Geometry check sheet. Reference: the model listing, model coordinates, mm. Give positions to 0.01 mm unless a question says otherwise; leave off trailing zeros. Loops run counter-clockwise (first coordinate to the right, second up) from the corner with the lowest first, then second, coordinate; pieces in that order, holes last.
1. Cross-section at D-D, the plane z = 76.5. Record the cut outline in (x, y).
2. Release check for a two-part mould opening along X. For faces 1 (the flat face through (64, 0, 54)), 2 (the cylindrical face through (36.71, 2.46, 91.41)), 3 (the flat face through (65.6, 2.5, -8.5)), 4 (the cylindrical face through (72.68, 2.54, 40.54)) record: +X half, -X half, draft (parallel to the pull), parting line (faces both ways), or undercut.
3. Go/stop test with flat-tipped pins: pin 1 Ø1.5 at (y, z) = (4, 19) entering from +X; pin 2 Ø3 at (x, y) = (39, 3.5) entering from +Z; pin 3 Ø3 at (x, y) = (58.5, 3.5) entering from +Z. Record where each tip stops, or that it passes through.
4. Cross-section at B-B, the plane x = 63.5. Record the cut outline in (y, z), plus the area to 3 significant figures.
5. Material ranges on L1, parallel to X at y = 3.7, z = 46.5; L2, parallel to X at y = 0.55, z = 43; L3, parallel to Z at x = 58, y = 3.75, recorded low to high.
6. Cross-section at C-C, the plane y = 2.35. Record the cut outline in (x, z), plus the area to 3 significant figures.
7. Cross-section at A-A, the plane z = 48. Record the cut outline in (x, y), plus the area to 3 significant figures.
from build123d import *

# Parameters (mm, degrees)
EXTRUDE_1_DEPTH     = 5
SKETCH_3_R          = 11
CUT_EXTRUDE_1_DEPTH = 158.534808963


with BuildPart() as part:
    # Эскиз1 → Вытянуть1 (new body)
    with BuildSketch(Plane(origin=(0, 0, 0), x_dir=(1, 0, 0), z_dir=(0, 1, 0))):
        with BuildLine():
            Line((110.693591381, -10.706034223), (86.987107148, -10.47450238))
            ThreePointArc((86.987107148, -10.47450238), (85.452697722, -10.217456373), (84.071576651, -9.501223505))
            Line((84.071576651, -9.501223505), (67.773001994, 2.498048819))
            ThreePointArc((67.773001994, 2.498048819), (66.350950932, 4.124659089), (65.74794659, 6.199382193))
            Line((65.74794659, 6.199382193), (65.441843699, 10.89653157))
            ThreePointArc((65.441843699, 10.89653157), (63.704749785, 14.369065402), (60.006376962, 15.55144645))
            ThreePointArc((60.006376962, 15.55144645), (38.518658839, -92.399615134), (114.99158645, -13.234944542))
            ThreePointArc((114.99158645, -13.234944542), (113.18036629, -11.396421777), (110.693591381, -10.706034223))
        make_face()
    extrude(amount=EXTRUDE_1_DEPTH)

    # Эскиз3 → Вырез-Вытянуть1 (cut, through all)
    with BuildSketch(Plane(origin=(0, 5, 0), x_dir=(1, 0, 0), z_dir=(0, 1, 0))):
        with Locations(Location((61.772466567, -41.971863474, 0), (0, 0, 270))):
            Circle(SKETCH_3_R)
    extrude(amount=-CUT_EXTRUDE_1_DEPTH, mode=Mode.SUBTRACT)


solid = part.part
Result:
1. outline: (19.62, 0) - (110.63, 0) - (110.63, 5) - (19.62, 5) - close
2. face 1: draft
2. face 2: parting line
2. face 3: +X half
2. face 4: undercut
3. pin 1: stops at x = 118.17
3. pin 2: stops at z = 93.39
3. pin 3: stops at z = 98.71
4. outline: (0, -14.54) - (5, -14.54) - (5, 31.11) - (0, 31.11) - close; (0, 52.84) - (5, 52.84) - (5, 98.92) - (0, 98.92) - close
4. area: 459 mm2
5. L1: x = 7.97 to 51.75, 71.8 to 122.27
5. L2: x = 7.78 to 50.82, 72.72 to 122.47
5. L3: z = -15.34 to 31.64, 52.3 to 98.5
6. outline: (60.01, -15.55) arc R5 ccw to (65.44, -10.9) - (65.75, -6.2) arc R5 cw to (67.77, -2.5) - (84.07, 9.5) arc R5 cw to (86.99, 10.47) - (110.69, 10.71) arc R5 ccw to (114.99, 13.23) arc R57.36 ccw (long way) to start; hole circle Ø22 at (61.77, 41.97)
6. area: 9,210 mm2
7. outline: (8.12, 0) - (52.57, 0) - (52.57, 5) - (8.12, 5) - close; (70.97, 0) - (122.12, 0) - (122.12, 5) - (70.97, 5) - close
7. area: 478 mm2
